Geometry: final body of the model. Coordinates: model frame, mm. Give positions to 0.01 mm unless a question says otherwise; leave off trailing zeros. Write each loop counter-clockwise with the first axis right and the second up, starting at its lowest first coordinate (ties: lowest second). Pieces come first, ordered by that corner, then holes.
Q1. Section A-A (x = 72). Return the cut outline in (y, z), plus the area to 3 significant figures.
Q2. Section C-C (x = -30). Return the cut outline in (y, z), plus the area to 3 significant figures.
Q3. Line query: line 1 (Y direction, x = 10, z = 5.75); line 2 (X direction, y = 120.5, z = 8.25); line 3 (X direction, y = 52, z = 3). Output: solid intervals per line, ascending.
Q4. Section B-B (y = 70). Return the cut outline in (x, z).
Q5. Mould query, pull axis Y, two halves, no side actions, for faces 1 (the cylindrical face through (30.33, 92.48, 4.93)), 2 (the flat face through (100.5, 73, 5)), 3 (the flat face through (50, 0, 5)). Classes: +Y half, -Y half, draft (parallel to the pull), parting line (faces both ways), or undercut.
Q6. Pin query (flat end, axial travel): pin 1 Ø5 at (x, z) = (70.5, 3) entering from -Y; pin 2 Ø4 at (x, y) = (30, 90) entering from +Z. Return the tip coordinate at first contact, or that it passes through.
Q7. Section D-D (y = 50). Return the cut outline in (x, z), plus the area to 3 significant figures.
from build123d import *

# Parameters (mm, degrees)
BOSS_EXTRUDE1_DEPTH = 10
CUT_EXTRUDE1_REACH  = 181.589
SKETCH3_R           = 19.25
SKETCH3_R_2         = 2.5
SKETCH3_R_3         = 2.885000751


with BuildPart() as part:
    # Sketch1 → Boss-Extrude1 (new body)
    with BuildSketch(Plane.XY):
        Polygon((0, 0), (100.5, 0), (100.5, 148.49893218), (-40, 148.49893218), (-40, 60), align=None)
    extrude(amount=BOSS_EXTRUDE1_DEPTH)

    # Sketch3 → Cut-Extrude1 (cut, up to next)
    with BuildSketch(Plane(origin=(0, 0, 0), x_dir=(-1, 0, 0), z_dir=(0, 0, -1)), mode=Mode.PRIVATE) as cut_extrude1_sk1:
        with Locations((-72, 119.99893218)):
            Circle(SKETCH3_R)
    cut_extrude1_tool1 = extrude(cut_extrude1_sk1.sketch, amount=-CUT_EXTRUDE1_REACH, mode=Mode.PRIVATE) & part.part
    # Sketch3 → Cut-Extrude1 (cut, up to next)
    with BuildSketch(Plane(origin=(0, 0, 0), x_dir=(-1, 0, 0), z_dir=(0, 0, -1)), mode=Mode.PRIVATE) as cut_extrude1_sk2:
        with Locations((-30, 50)):
            Circle(SKETCH3_R_2)
    cut_extrude1_tool2 = extrude(cut_extrude1_sk2.sketch, amount=-CUT_EXTRUDE1_REACH, mode=Mode.PRIVATE) & part.part
    # Sketch3 → Cut-Extrude1 (cut, up to next)
    with BuildSketch(Plane(origin=(0, 0, 0), x_dir=(-1, 0, 0), z_dir=(0, 0, -1)), mode=Mode.PRIVATE) as cut_extrude1_sk3:
        with Locations((-10, 50)):
            Circle(SKETCH3_R_2)
    cut_extrude1_tool3 = extrude(cut_extrude1_sk3.sketch, amount=-CUT_EXTRUDE1_REACH, mode=Mode.PRIVATE) & part.part
    # Sketch3 → Cut-Extrude1 (cut, up to next)
    with BuildSketch(Plane(origin=(0, 0, 0), x_dir=(-1, 0, 0), z_dir=(0, 0, -1)), mode=Mode.PRIVATE) as cut_extrude1_sk4:
        with Locations((-30, 10)):
            Circle(SKETCH3_R_2)
    cut_extrude1_tool4 = extrude(cut_extrude1_sk4.sketch, amount=-CUT_EXTRUDE1_REACH, mode=Mode.PRIVATE) & part.part
    # Sketch3 → Cut-Extrude1 (cut, up to next)
    with BuildSketch(Plane(origin=(0, 0, 0), x_dir=(-1, 0, 0), z_dir=(0, 0, -1)), mode=Mode.PRIVATE) as cut_extrude1_sk5:
        with Locations((-10, 10)):
            Circle(SKETCH3_R_2)
    cut_extrude1_tool5 = extrude(cut_extrude1_sk5.sketch, amount=-CUT_EXTRUDE1_REACH, mode=Mode.PRIVATE) & part.part
    # Sketch3 → Cut-Extrude1 (cut, up to next)
    with BuildSketch(Plane(origin=(0, 0, 0), x_dir=(-1, 0, 0), z_dir=(0, 0, -1)), mode=Mode.PRIVATE) as cut_extrude1_sk6:
        with Locations((30, 70)):
            Circle(SKETCH3_R_2)
    cut_extrude1_tool6 = extrude(cut_extrude1_sk6.sketch, amount=-CUT_EXTRUDE1_REACH, mode=Mode.PRIVATE) & part.part
    # Sketch3 → Cut-Extrude1 (cut, up to next)
    with BuildSketch(Plane(origin=(0, 0, 0), x_dir=(-1, 0, 0), z_dir=(0, 0, -1)), mode=Mode.PRIVATE) as cut_extrude1_sk7:
        with Locations((30, 90)):
            Circle(SKETCH3_R_2)
    cut_extrude1_tool7 = extrude(cut_extrude1_sk7.sketch, amount=-CUT_EXTRUDE1_REACH, mode=Mode.PRIVATE) & part.part
    # Sketch3 → Cut-Extrude1 (cut, up to next)
    with BuildSketch(Plane(origin=(0, 0, 0), x_dir=(-1, 0, 0), z_dir=(0, 0, -1)), mode=Mode.PRIVATE) as cut_extrude1_sk8:
        with Locations((10, 90)):
            Circle(SKETCH3_R_2)
    cut_extrude1_tool8 = extrude(cut_extrude1_sk8.sketch, amount=-CUT_EXTRUDE1_REACH, mode=Mode.PRIVATE) & part.part
    # Sketch3 → Cut-Extrude1 (cut, up to next)
    with BuildSketch(Plane(origin=(0, 0, 0), x_dir=(-1, 0, 0), z_dir=(0, 0, -1)), mode=Mode.PRIVATE) as cut_extrude1_sk9:
        with Locations((10, 70)):
            Circle(SKETCH3_R_2)
    cut_extrude1_tool9 = extrude(cut_extrude1_sk9.sketch, amount=-CUT_EXTRUDE1_REACH, mode=Mode.PRIVATE) & part.part
    # Sketch3 → Cut-Extrude1 (cut, up to next)
    with BuildSketch(Plane(origin=(0, 0, 0), x_dir=(-1, 0, 0), z_dir=(0, 0, -1)), mode=Mode.PRIVATE) as cut_extrude1_sk10:
        with Locations((-10, 70)):
            Circle(SKETCH3_R_2)
    cut_extrude1_tool10 = extrude(cut_extrude1_sk10.sketch, amount=-CUT_EXTRUDE1_REACH, mode=Mode.PRIVATE) & part.part
    # Sketch3 → Cut-Extrude1 (cut, up to next)
    with BuildSketch(Plane(origin=(0, 0, 0), x_dir=(-1, 0, 0), z_dir=(0, 0, -1)), mode=Mode.PRIVATE) as cut_extrude1_sk11:
        with Locations((-10, 90)):
            Circle(SKETCH3_R_2)
    cut_extrude1_tool11 = extrude(cut_extrude1_sk11.sketch, amount=-CUT_EXTRUDE1_REACH, mode=Mode.PRIVATE) & part.part
    # Sketch3 → Cut-Extrude1 (cut, up to next)
    with BuildSketch(Plane(origin=(0, 0, 0), x_dir=(-1, 0, 0), z_dir=(0, 0, -1)), mode=Mode.PRIVATE) as cut_extrude1_sk12:
        with Locations((-30, 90)):
            Circle(SKETCH3_R_2)
    cut_extrude1_tool12 = extrude(cut_extrude1_sk12.sketch, amount=-CUT_EXTRUDE1_REACH, mode=Mode.PRIVATE) & part.part
    # Sketch3 → Cut-Extrude1 (cut, up to next)
    with BuildSketch(Plane(origin=(0, 0, 0), x_dir=(-1, 0, 0), z_dir=(0, 0, -1)), mode=Mode.PRIVATE) as cut_extrude1_sk13:
        with Locations((-30, 70)):
            Circle(SKETCH3_R_2)
    cut_extrude1_tool13 = extrude(cut_extrude1_sk13.sketch, amount=-CUT_EXTRUDE1_REACH, mode=Mode.PRIVATE) & part.part
    # Sketch3 → Cut-Extrude1 (cut, up to next)
    with BuildSketch(Plane(origin=(0, 0, 0), x_dir=(-1, 0, 0), z_dir=(0, 0, -1)), mode=Mode.PRIVATE) as cut_extrude1_sk14:
        with Locations((-95.5, 143.49893218)):
            Circle(SKETCH3_R_3)
    cut_extrude1_tool14 = extrude(cut_extrude1_sk14.sketch, amount=-CUT_EXTRUDE1_REACH, mode=Mode.PRIVATE) & part.part
    # Sketch3 → Cut-Extrude1 (cut, up to next)
    with BuildSketch(Plane(origin=(0, 0, 0), x_dir=(-1, 0, 0), z_dir=(0, 0, -1)), mode=Mode.PRIVATE) as cut_extrude1_sk15:
        with Locations((-48.5, 143.49893218)):
            Circle(SKETCH3_R_3)
    cut_extrude1_tool15 = extrude(cut_extrude1_sk15.sketch, amount=-CUT_EXTRUDE1_REACH, mode=Mode.PRIVATE) & part.part
    # Sketch3 → Cut-Extrude1 (cut, up to next)
    with BuildSketch(Plane(origin=(0, 0, 0), x_dir=(-1, 0, 0), z_dir=(0, 0, -1)), mode=Mode.PRIVATE) as cut_extrude1_sk16:
        with Locations((-48.5, 96.49893218)):
            Circle(SKETCH3_R_3)
    cut_extrude1_tool16 = extrude(cut_extrude1_sk16.sketch, amount=-CUT_EXTRUDE1_REACH, mode=Mode.PRIVATE) & part.part
    # Sketch3 → Cut-Extrude1 (cut, up to next)
    with BuildSketch(Plane(origin=(0, 0, 0), x_dir=(-1, 0, 0), z_dir=(0, 0, -1)), mode=Mode.PRIVATE) as cut_extrude1_sk17:
        with Locations((-95.5, 96.49893218)):
            Circle(SKETCH3_R_3)
    cut_extrude1_tool17 = extrude(cut_extrude1_sk17.sketch, amount=-CUT_EXTRUDE1_REACH, mode=Mode.PRIVATE) & part.part
    add(cut_extrude1_tool1.solids().sort_by_distance((72, 119.998932, 0))[0], mode=Mode.SUBTRACT)
    add(cut_extrude1_tool2.solids().sort_by_distance((30, 50, 0))[0], mode=Mode.SUBTRACT)
    add(cut_extrude1_tool3.solids().sort_by_distance((10, 50, 0))[0], mode=Mode.SUBTRACT)
    add(cut_extrude1_tool4.solids().sort_by_distance((30, 10, 0))[0], mode=Mode.SUBTRACT)
    add(cut_extrude1_tool5.solids().sort_by_distance((10, 10, 0))[0], mode=Mode.SUBTRACT)
    add(cut_extrude1_tool6.solids().sort_by_distance((-30, 70, 0))[0], mode=Mode.SUBTRACT)
    add(cut_extrude1_tool7.solids().sort_by_distance((-30, 90, 0))[0], mode=Mode.SUBTRACT)
    add(cut_extrude1_tool8.solids().sort_by_distance((-10, 90, 0))[0], mode=Mode.SUBTRACT)
    add(cut_extrude1_tool9.solids().sort_by_distance((-10, 70, 0))[0], mode=Mode.SUBTRACT)
    add(cut_extrude1_tool10.solids().sort_by_distance((10, 70, 0))[0], mode=Mode.SUBTRACT)
    add(cut_extrude1_tool11.solids().sort_by_distance((10, 90, 0))[0], mode=Mode.SUBTRACT)
    add(cut_extrude1_tool12.solids().sort_by_distance((30, 90, 0))[0], mode=Mode.SUBTRACT)
    add(cut_extrude1_tool13.solids().sort_by_distance((30, 70, 0))[0], mode=Mode.SUBTRACT)
    add(cut_extrude1_tool14.solids().sort_by_distance((95.5, 143.498932, 0))[0], mode=Mode.SUBTRACT)
    add(cut_extrude1_tool15.solids().sort_by_distance((48.5, 143.498932, 0))[0], mode=Mode.SUBTRACT)
    add(cut_extrude1_tool16.solids().sort_by_distance((48.5, 96.498932, 0))[0], mode=Mode.SUBTRACT)
    add(cut_extrude1_tool17.solids().sort_by_distance((95.5, 96.498932, 0))[0], mode=Mode.SUBTRACT)


solid = part.part
Computed:
1. outline: (0, 0) - (100.75, 0) - (100.75, 10) - (0, 10) - close; (139.25, 0) - (148.5, 0) - (148.5, 10) - (139.25, 10) - close
1. area: 1,100 mm2
2. outline: (45, 0) - (67.5, 0) - (67.5, 10) - (45, 10) - close; (72.5, 0) - (87.5, 0) - (87.5, 10) - (72.5, 10) - close; (92.5, 0) - (148.5, 0) - (148.5, 10) - (92.5, 10) - close
2. area: 935 mm2
3. line 1: y = 0 to 7.5, 12.5 to 47.5, 52.5 to 67.5, 72.5 to 87.5, 92.5 to 148.5
3. line 2: x = -40 to 52.76, 91.24 to 100.5
3. line 3: x = -34.67 to 8.5, 11.5 to 28.5, 31.5 to 100.5
4. outline: (-40, 0) - (-32.5, 0) - (-32.5, 10) - (-40, 10) - close; (-27.5, 0) - (-12.5, 0) - (-12.5, 10) - (-27.5, 10) - close; (-7.5, 0) - (7.5, 0) - (7.5, 10) - (-7.5, 10) - close; (12.5, 0) - (27.5, 0) - (27.5, 10) - (12.5, 10) - close; (32.5, 0) - (100.5, 0) - (100.5, 10) - (32.5, 10) - close
5. face 1: undercut
5. face 2: draft
5. face 3: -Y half
6. pin 1: stops at y = 0
6. pin 2: passes through
7. outline: (-33.33, 0) - (7.5, 0) - (7.5, 10) - (-33.33, 10) - close; (12.5, 0) - (27.5, 0) - (27.5, 10) - (12.5, 10) - close; (32.5, 0) - (100.5, 0) - (100.5, 10) - (32.5, 10) - close
7. area: 1,240 mm2
